Part model, mm, in its own coordinate system. A direction names the side the tool comes from. Coordinates: 2 decimals unless noted, no trailing zeros. Loops run counter-clockwise (first coordinate to the right, second up) from the corner with the lowest first, then second, coordinate; pieces in that order, holes last. Notation, with made-up numbers: (68.5, 66) - (77.5, 66) arc R21 ccw to (77.5, 77) - close; hole circle Ø3 at (72.5, 45.5). An arc over 180 degrees is marked (long way). Use a Markdown table: item, result. Add a question column.
1. Band-saw the part on B-B, the plane x = -13.75. Give the cut face in (y, z).
2. Band-saw the part on A-A, the plane y = 1. Give the cut face in (x, z).
3. Pull direction X, two halves, no side cores. Call faces 1 (the flat face through (2, 0, -1.5)), 2 (the flat face through (-7.04, -0.042, -0.773)), 3 (the cylindrical face through (-2.975, 0.042, -1.668)), 4 (the cylindrical face through (-1.5, 0.07, -0.02)): pulls with the +X half, pulls with the -X half, needs draft (parallel to the pull), parting line crosses it, or undercut.
4. Band-saw the part on D-D, the plane y = -2. Give the cut face in (x, z), plus the area to 3 significant figures.
5. Wall check: probe 1 along Y at (x, z) = (0, -0.4); probe 2 along Z at (x, y) = (0.75, 2.25); probe 3 along Z at (x, y) = (-14.5, 2.25). Give the ranges that are in metal, low to high. Write a range as [from, to].
6. Drop flat-ended pins along their axis: pin 1 (2 mm diameter, centred on y = -2.5, z = -4.5, fed in from +X); pin 2 (2 mm diameter, centred on y = 2.5, z = 0.5, fed in from -X); pin 3 (1 mm diameter, centred on y = 1.5, z = -3.5, fed in from +X); pin 4 (1.8 mm diameter, centred on x = 0, y = 0, fed in from +Z). Give the stop position or say it passes through.
7. Band-saw the part on C-C, the plane z = 0.25. Give the cut face in (x, y), plus the area to 3 significant figures.
8. 3-axis set-ups, long thin cutter, end or side, ignore diameter. For faces 5 (the flat face through (-6.96, -0.042, -3.727)), 6 (the flat face through (-16, 0, -3)): which of +Z, -Z, +X, -X, +Y, -Y reach the whole face in a straight line?
from build123d import *

# Parameters (mm, degrees)
BOSS_EXTRUDE1_DEPTH      = 3
BOSS_EXTRUDE1_DEPTH_BACK = 3
CUT_EXTRUDE1_DEPTH       = 3
CUT_EXTRUDE1_DEPTH_BACK  = 3
SKETCH2_R                = 1.5
CUT_EXTRUDE3_DEPTH       = 3
CUT_EXTRUDE3_DEPTH_BACK  = 3
SKETCH4_R                = 1.5
FILLET1_R                = 5


with BuildPart() as part:
    # Sketch3 → Boss-Extrude1 (new, two sides: drawn at the far end of the back side and taken through both)
    with BuildSketch(Plane(origin=(0, 0, 0), x_dir=(1, 0, 0), z_dir=(0, 1, 0)).offset(-BOSS_EXTRUDE1_DEPTH_BACK)):
        Polygon((-3, -1.5), (3, -1.5), (3, 1.5), (-3, 1.5), (-11, 6), (-17, 6), (-17, 3), (-11, 3), align=None)
    extrude(amount=BOSS_EXTRUDE1_DEPTH + BOSS_EXTRUDE1_DEPTH_BACK)

    # Sketch2 → Cut-Extrude1 (cut, two sides: drawn at the far end of the back side and taken through both)
    with BuildSketch(Plane.XY.offset(-CUT_EXTRUDE1_DEPTH_BACK)):
        with BuildLine():
            ThreePointArc((0, 3), (2.121320344, 2.121320344), (3, 0))
            Line((3, 0), (3, 3))
            Line((3, 3), (0, 3))
        make_face()
        with BuildLine():
            ThreePointArc((3, 0), (2.121320338, -2.121320349), (-1.5e-08, -3))
            Line((-1.5e-08, -3), (3, -3))
            Line((3, -3), (3, 0))
        make_face()
        Circle(SKETCH2_R)
    extrude(amount=CUT_EXTRUDE1_DEPTH + CUT_EXTRUDE1_DEPTH_BACK, mode=Mode.SUBTRACT)

    # Sketch4 → Cut-Extrude3 (cut, two sides: drawn at the far end of the back side and taken through both)
    with BuildSketch(Plane.XY.offset(-3).offset(-CUT_EXTRUDE3_DEPTH_BACK)):
        with BuildLine():
            ThreePointArc((-14, -3), (-16.121320333, -2.121320355), (-17, -3.1e-08))
            Line((-17, -3.1e-08), (-17, -3))
            Line((-17, -3), (-14, -3))
        make_face()
        with BuildLine():
            ThreePointArc((-17, -3.1e-08), (-16.121320355, 2.121320333), (-14, 3))
            Line((-14, 3), (-17, 3))
            Line((-17, 3), (-17, -3.1e-08))
        make_face()
        with Locations((-14, 0)):
            Circle(SKETCH4_R)
    extrude(amount=CUT_EXTRUDE3_DEPTH + CUT_EXTRUDE3_DEPTH_BACK, mode=Mode.SUBTRACT)

    # Fillet1
    fillet1_edges = [part.edges().sort_by_distance(p)[0] for p in [
        (-3, 0, -1.5),
        (-3, 0, 1.5),
        (-11, 0, -3),
        (-11, 0, -6),
    ]]
    fillet(fillet1_edges, radius=FILLET1_R)


solid = part.part
Geometry check:
| question | item | result |
|---|---|---|
| 1 | outline | (-3, -6) - (-1.48, -6) - (-1.48, -3) - (-3, -3) - close; (1.48, -6) - (3, -6) - (3, -3) - (1.48, -3) - close |
| 2 | outline | (-16.83, -6) - (-15.12, -6) - (-15.12, -3) - (-16.83, -3) - close; (-12.88, -6) - (-12.31, -6) arc R5 ccw to (-9.86, -5.36) - (-4.14, -2.14) arc R5 cw to (-1.69, -1.5) - (-1.12, -1.5) - (-1.12, 1.5) - (-1.69, 1.5) arc R5 ccw to (-4.14, 0.86) - (-9.86, -2.36) arc R5 cw to (-12.31, -3) - (-12.88, -3) - close; (1.12, -1.5) - (2.83, -1.5) - (2.83, 1.5) - (1.12, 1.5) - close |
| 3 | face 1 | needs draft |
| 3 | face 2 | pulls with the -X half |
| 3 | face 3 | pulls with the +X half |
| 3 | face 4 | undercut |
| 4 | outline | (-16.24, -6) - (-12.31, -6) arc R5 ccw to (-9.86, -5.36) - (-4.14, -2.14) arc R5 cw to (-1.69, -1.5) - (2.24, -1.5) - (2.24, 1.5) - (-1.69, 1.5) arc R5 ccw to (-4.14, 0.86) - (-9.86, -2.36) arc R5 cw to (-12.31, -3) - (-16.24, -3) - close |
| 4 | area | 55.4 mm^2 |
| 5 | probe 1 | y = [-3, -1.5], [1.5, 3] |
| 5 | probe 2 | z = [-1.5, 1.5] |
| 5 | probe 3 | z = [-6, -3] |
| 6 | pin 1 | stops at x = -6.56 |
| 6 | pin 2 | stops at x = -6.56 |
| 6 | pin 3 | stops at x = -5.67 |
| 6 | pin 4 | passes through |
| 7 | outline | (-5.22, -3) - (0, -3) arc R3 ccw to (0, 3) - (-5.22, 3) - close; hole circle Ø3 at (0, 0) |
| 7 | area | 38.4 mm^2 |
| 8 | face 5 | -Z, +X, +Y, -Y |
| 8 | face 6 | +Z, -X, +Y, -Y |
